```python
from build123d import *

# Parameters (mm, degrees)
F0_W     = 37
F0_H     = 37
F0_W_2   = 33
F0_H_2   = 33
F1_DEPTH = 9
F2_W     = 37
F2_H     = 37
F3_DEPTH = 1.5
F5_DEPTH = 9
F7_D     = 5


with BuildPart() as f1:
    # F0 (on Front) → F1 (new body)
    with BuildSketch(Plane.XZ):
        with Locations((18.5, 18.5)):
            Rectangle(F0_W, F0_H)
        with Locations((18.5, 18.5)):
            Rectangle(F0_W_2, F0_H_2, mode=Mode.SUBTRACT)
    extrude(amount=F1_DEPTH)

    # F2 (on face) → F3 (join)
    with BuildSketch(Plane(origin=(0, 0, 0), x_dir=(-1, 0, 0), z_dir=(0, 1, 0))):
        with Locations((-18.5, 18.5)):
            Rectangle(F2_W, F2_H)
    extrude(amount=F3_DEPTH)

    # F4 (on face) → F5 (join, through all)
    with BuildSketch(Plane.XZ.offset(9)):
        Polygon((23.5, 35), (13.5, 35), (14.5, 33.294015), (22.5, 33.294015), align=None)
        Polygon((14.5, 3.705985), (13.5, 2), (23.5, 2), (22.5, 3.705985), align=None)
    extrude(amount=-F5_DEPTH)

    # F7 (through all)
    with Locations(Plane.XZ):
        with Locations((18.5, 18.5)):
            Hole(F7_D / 2)


solid = f1.part
```
Work out the finished part from the listing and answer in its coordinate system (mm). A direction names the side the tool comes from. Coordinates: 2 decimals unless noted, no trailing zeros. Loops run counter-clockwise (first coordinate to the right, second up) from the corner with the lowest first, then second, coordinate; pieces in that order, holes last.
1) For a pull along X with two mould halves and no side action, classify faces 1 (the flat face through (8, -4, 2)), 2 (the flat face through (37, -4, 18)), 3 (the flat face through (0, -4, 18)), 4 (the flat face through (14.007, -4.563, 2.865)) as +X half, -X half, draft (parallel to the pull), parting line (faces both ways), or undercut.
Results:
face 1: undercut
face 2: +X half
face 3: -X half
face 4: undercut
2) Section C-C (y = -5.25) is taken. Give the vertices of the cut face in (x, z), plus the area to 3 significant figures.
Results:
outline: (0, 0) - (37, 0) - (37, 37) - (0, 37) - close; hole (2, 2) - (13.5, 2) - (14.5, 3.71) - (22.5, 3.71) - (23.5, 2) - (35, 2) - (35, 35) - (23.5, 35) - (22.5, 33.29) - (14.5, 33.29) - (13.5, 35) - (2, 35) - close
area: 311 mm2
3) Section A-A (z = 16.5) is taken. Give the vertices of the cut face in (x, y), plus the area to 3 significant figures.
Results:
outline: (0, -9) - (2, -9) - (2, 0) - (17, 0) - (17, 1.5) - (0, 1.5) - close; (20, 0) - (35, 0) - (35, -9) - (37, -9) - (37, 1.5) - (20, 1.5) - close
area: 87.0 mm2
4) For faces 5 (the flat face through (23, 1.5, 19)), 6 (the flat face through (18, -5, 33.294)), determine the directions among +Z, -Z, +X, -X, +Y, -Y from which every point of the face is accessible in a straight line to the end or side of a thin tool.
Results:
face 5: +Z, -Z, +X, -X, +Y
face 6: -Y
5) Consider probe 1 along X at (y, z) = (-8.5, 16); probe 2 along Z at (x, y) = (18.5, 1). Determine where each line is inside the solid, lowest interval first.
Results:
probe 1: x = 0 to 2, 35 to 37
probe 2: z = 0 to 16, 21 to 37
6) Section D-D (x = 27.5) is taken. Give the vertices of the cut face in (y, z), plus the area to 3 significant figures.
Results:
outline: (-9, 0) - (1.5, 0) - (1.5, 37) - (-9, 37) - (-9, 35) - (0, 35) - (0, 2) - (-9, 2) - close
area: 91.5 mm2
7) Section B-B (x = 18.5) is taken. Give the vertices of the cut face in (y, z).
Results:
outline: (-9, 0) - (1.5, 0) - (1.5, 16) - (0, 16) - (0, 3.71) - (-9, 3.71) - close; (-9, 33.29) - (0, 33.29) - (0, 21) - (1.5, 21) - (1.5, 37) - (-9, 37) - close
